Source: CAD feature listing. Evaluate the final solid. Frame: model axes, mm. A direction names the side the tool comes from. Give positions to 0.01 mm unless a question says otherwise; leave off trailing zeros. Order: outer loops, then holes, each group sorted by start corner. A loop starts at its lowest first (then second) coordinate and runs counter-clockwise, first axis right, second up. Notation, with made-up numbers: (8, 82.5) - (49, 82.5) arc R34 ccw to (49, 119.5) - close; hole circle Ø8 at (58, -2). An arc over 180 degrees is marked (long way). Answer as CSV lines item,"result".
```python
from build123d import *

# Parameters (mm, degrees)
IZIM1_R                     = 3.4
IZIM1_R_2                   = 2.5
Y_KSEKLIK_EKSTR_ZYON1_DEPTH = 80
FILLET1_R                   = 2


with BuildPart() as part:
    # Çizim1 → Yükseklik-Ekstrüzyon1 (new body)
    with BuildSketch(Plane.XY):
        with BuildLine():
            Line((18.25, 0), (30, 0))
            Line((30, 0), (30, -11.75))
            Line((30, -11.75), (27.5, -11.75))
            Line((27.5, -11.75), (27.5, -9.75))
            Line((27.5, -9.75), (21.463651766, -9.75))
            ThreePointArc((21.463651766, -9.75), (19.5, -15), (21.463651766, -20.25))
            Line((21.463651766, -20.25), (27.5, -20.25))
            Line((27.5, -20.25), (27.5, -18.25))
            Line((27.5, -18.25), (30, -18.25))
            Line((30, -18.25), (30, -30))
            Line((30, -30), (18.25, -30))
            Line((18.25, -30), (18.25, -27.5))
            Line((18.25, -27.5), (20.25, -27.5))
            Line((20.25, -27.5), (20.25, -21.463651766))
            ThreePointArc((20.25, -21.463651766), (15, -19.5), (9.75, -21.463651766))
            Line((9.75, -21.463651766), (9.75, -27.5))
            Line((9.75, -27.5), (11.75, -27.5))
            Line((11.75, -27.5), (11.75, -30))
            Line((11.75, -30), (0, -30))
            ThreePointArc((0, -30), (-21.213203436, -21.213203436), (-30, 0))
            Line((-30, 0), (-30, 11.75))
            Line((-30, 11.75), (-27.5, 11.75))
            Line((-27.5, 11.75), (-27.5, 9.75))
            Line((-27.5, 9.75), (-21.463651766, 9.75))
            ThreePointArc((-21.463651766, 9.75), (-19.5, 15), (-21.463651766, 20.25))
            Line((-21.463651766, 20.25), (-27.5, 20.25))
            Line((-27.5, 20.25), (-27.5, 18.25))
            Line((-27.5, 18.25), (-30, 18.25))
            Line((-30, 18.25), (-30, 30))
            Line((-30, 30), (-18.25, 30))
            Line((-18.25, 30), (-18.25, 27.5))
            Line((-18.25, 27.5), (-20.25, 27.5))
            Line((-20.25, 27.5), (-20.25, 21.463651766))
            ThreePointArc((-20.25, 21.463651766), (-15, 19.5), (-9.75, 21.463651766))
            Line((-9.75, 21.463651766), (-9.75, 27.5))
            Line((-9.75, 27.5), (-11.75, 27.5))
            Line((-11.75, 27.5), (-11.75, 30))
            Line((-11.75, 30), (0, 30))
            Line((0, 30), (0, 18.25))
            Line((0, 18.25), (-2.5, 18.25))
            Line((-2.5, 18.25), (-2.5, 20.25))
            Line((-2.5, 20.25), (-8.536348234, 20.25))
            ThreePointArc((-8.536348234, 20.25), (-10.5, 15), (-8.536348234, 9.75))
            Line((-8.536348234, 9.75), (-2.5, 9.75))
            Line((-2.5, 9.75), (-2.5, 11.75))
            Line((-2.5, 11.75), (0, 11.75))
            Line((0, 11.75), (0, 8.85))
            ThreePointArc((0, 8.85), (-6.257895014, -6.257895014), (8.85, 0))
            Line((8.85, 0), (11.75, 0))
            Line((11.75, 0), (11.75, -2.5))
            Line((11.75, -2.5), (9.75, -2.5))
            Line((9.75, -2.5), (9.75, -8.536348234))
            ThreePointArc((9.75, -8.536348234), (15, -10.5), (20.25, -8.536348234))
            Line((20.25, -8.536348234), (20.25, -2.5))
            Line((20.25, -2.5), (18.25, -2.5))
            Line((18.25, -2.5), (18.25, 0))
        make_face()
        with Locations((25.125, -4.875)):
            Circle(IZIM1_R, mode=Mode.SUBTRACT)
        with Locations((25.125, -25.125)):
            Circle(IZIM1_R, mode=Mode.SUBTRACT)
        with Locations((15, -15)):
            Circle(IZIM1_R_2, mode=Mode.SUBTRACT)
        with Locations((-14.849242405, -14.849242405)):
            Circle(IZIM1_R_2, mode=Mode.SUBTRACT)
        with Locations((-4.875, 25.125)):
            Circle(IZIM1_R, mode=Mode.SUBTRACT)
        with Locations((-25.125, 25.125)):
            Circle(IZIM1_R, mode=Mode.SUBTRACT)
        with Locations((-15, 15)):
            Circle(IZIM1_R_2, mode=Mode.SUBTRACT)
        with BuildLine():
            Line((-17.382505973, -18.796719535), (-18.651386187, -20.065599749))
            ThreePointArc((-18.651386187, -20.065599749), (-18.943614734, -20.809160633), (-18.597987217, -21.529453581))
            ThreePointArc((-18.597987217, -21.529453581), (-9.921933925, -26.663790563), (0, -28.45))
            Line((0, -28.45), (7.2, -28.45))
            ThreePointArc((7.2, -28.45), (7.907106781, -28.157106781), (8.2, -27.45))
            Line((8.2, -27.45), (8.2, -20.611577633))
            ThreePointArc((8.2, -20.611577633), (8.256120646, -20.281287208), (8.41818353, -19.988069007))
            ThreePointArc((8.41818353, -19.988069007), (10.119864462, -14.164129468), (7.244983946, -8.820998197))
            ThreePointArc((7.244983946, -8.820998197), (6.652264712, -8.594274715), (6.042451121, -8.769907893))
            ThreePointArc((6.042451121, -8.769907893), (-0.050937117, -10.649878188), (-6.126063635, -8.711707315))
            ThreePointArc((-6.126063635, -8.711707315), (-6.787438159, -8.533426454), (-7.408387658, -8.822601221))
            Line((-7.408387658, -8.822601221), (-10.901765275, -12.315978837))
            ThreePointArc((-10.901765275, -12.315978837), (-11.173564806, -12.818775974), (-11.125575276, -13.388316975))
            ThreePointArc((-11.125575276, -13.388316975), (-12.02081528, -17.67766953), (-16.310167834, -18.572909534))
            ThreePointArc((-16.310167834, -18.572909534), (-16.879708835, -18.524920004), (-17.382505973, -18.796719535))
        make_face(mode=Mode.SUBTRACT)
        with BuildLine():
            Line((-12.315978837, -10.901765275), (-8.822601221, -7.408387658))
            ThreePointArc((-8.822601221, -7.408387658), (-8.533426454, -6.787438159), (-8.711707315, -6.126063635))
            ThreePointArc((-8.711707315, -6.126063635), (-10.649878188, -0.050937117), (-8.769907893, 6.042451121))
            ThreePointArc((-8.769907893, 6.042451121), (-8.594274715, 6.652264712), (-8.820998197, 7.244983946))
            ThreePointArc((-8.820998197, 7.244983946), (-14.164129468, 10.119864462), (-19.988069007, 8.41818353))
            ThreePointArc((-19.988069007, 8.41818353), (-20.281287208, 8.256120646), (-20.611577633, 8.2))
            Line((-20.611577633, 8.2), (-27.45, 8.2))
            ThreePointArc((-27.45, 8.2), (-28.157106781, 7.907106781), (-28.45, 7.2))
            Line((-28.45, 7.2), (-28.45, 0))
            ThreePointArc((-28.45, 0), (-26.663790563, -9.921933925), (-21.529453581, -18.597987217))
            ThreePointArc((-21.529453581, -18.597987217), (-20.809160633, -18.943614734), (-20.065599749, -18.651386187))
            Line((-20.065599749, -18.651386187), (-18.796719535, -17.382505973))
            ThreePointArc((-18.796719535, -17.382505973), (-18.524920004, -16.879708835), (-18.572909534, -16.310167834))
            ThreePointArc((-18.572909534, -16.310167834), (-17.67766953, -12.02081528), (-13.388316975, -11.125575276))
            ThreePointArc((-13.388316975, -11.125575276), (-12.818775974, -11.173564806), (-12.315978837, -10.901765275))
        make_face(mode=Mode.SUBTRACT)
    extrude(amount=Y_KSEKLIK_EKSTR_ZYON1_DEPTH)

    # Fillet1
    fillet1_edges = [part.edges().sort_by_distance(p)[0] for p in [
        (-30, 30, 40),
        (0, 30, 40),
        (30, 0, 40),
        (30, -30, 40),
    ]]
    fillet(fillet1_edges, radius=FILLET1_R)


solid = part.part
```
(1) Cut plane A-A (x = 15). Return loops of the section in (y, z), then the cut area to 3 significant figures.
Completed:
outline,"(-19.5, 0) - (-17.5, 0) - (-17.5, 80) - (-19.5, 80) - close; (-12.5, 0) - (-10.5, 0) - (-10.5, 80) - (-12.5, 80) - close"
area,"320 mm²"
(2) Ray query, line 1 (Y direction, x = 15, z = 43.5); line 2 (X direction, y = 26.5, z = 36.5); line 3 (X direction, y = -9.5, z = 76). Return the intervals inside material, ascending. Write a range as from..to.
Completed:
line 1,"-19.5..-17.5, -12.5..-10.5"
line 2,"-30..-28.23, -22.02..-20.25, -9.75..-7.98, -1.77..0"
line 3,"-28.46..-26.82, -10.91..-8.09, -4.81..4.81, 7.97..11.13, 18.87..30"
(3) Cut plane D-D (z = 70). Give the number of separate pieces and of enclosed holes in the cut face, then the cut area to 3 significant figures.
Completed:
separate pieces,"1"
enclosed holes,"9"
area,"742 mm²"
(4) Cut plane C-C (x = -23). Return loops of the section in (y, z).
Completed:
outline,"(-19.26, 0) - (-16.75, 0) - (-16.75, 80) - (-19.26, 80) - close; (8.2, 0) - (9.75, 0) - (9.75, 80) - (8.2, 80) - close; (20.25, 0) - (22.47, 0) - (22.47, 80) - (20.25, 80) - close; (27.78, 0) - (30, 0) - (30, 80) - (27.78, 80) - close"
(5) Access query for faces 1 (the flat face through (-1, 11.75, 39)), 2 (the flat face through (-11, 27.5, 39)), 3 (the flat face through (11.75, -1, 39)). Directions: +Z, -Z, +X, -X, +Y, -Y. A direction counts if a zero-diameter tool reaches every point of the face in a straight line with its end or side. Return the directions, or none.
Completed:
face 1,"+Z, -Z, +X"
face 2,"+Z, -Z"
face 3,"+Z, -Z, +Y"
(6) Cut plane B-B (x = -15). Return loops of the section in (y, z).
Completed:
outline,"(-25.98, 0) - (-24.17, 0) - (-24.17, 80) - (-25.98, 80) - close; (-18.85, 0) - (-17.34, 0) - (-17.34, 80) - (-18.85, 80) - close; (-12.35, 0) - (-10.85, 0) - (-10.85, 80) - (-12.35, 80) - close; (10.16, 0) - (12.5, 0) - (12.5, 80) - (10.16, 80) - close; (17.5, 0) - (19.5, 0) - (19.5, 80) - (17.5, 80) - close"
(7) Mould query, pull axis Y, two halves, no side actions, for faces 4 (the flat face through (18.25, -1, 39)), 5 (the flat face through (-1, 18.25, 39)), 6 (the flat face through (-7, 30, 39)). Classes: released by +Y, released by -Y, zero draft, split by the parting line, or undercut.
Completed:
face 4,"zero draft"
face 5,"undercut"
face 6,"released by +Y"
(8) Contact query for flat-ended pins moving along their axis: pin 1 (5.5 mm diameter, centred on x = -23, z = 57, fed in from -Y); pin 2 (6.5 mm diameter, centred on x = -5.5, z = 37.5, fed in from -Y); pin 3 (6 mm diameter, centred on x = 4, z = 22.5, fed in from +Y) (3 decimals). Output: stop coordinate, or through.
Completed:
pin 1,"y = -22.13"
pin 2,"y = -29.92"
pin 3,"y = -5.415"
